```python
from build123d import *

# Parameters (mm, degrees)
F0_W     = 30
F0_H     = 50
F1_DEPTH = 25
F2_W     = 19.697615
F2_H     = 4.146867
F2_W_2   = 19.52483
F2_H_2   = 5.874727
F3_DEPTH = 10
F4_DEPTH = 10
F5_DEPTH = 25
F6_DEPTH = 25
F7_R     = 1.5
F2_R     = 3.544564
F8_DEPTH = 25


with BuildPart() as f1:
    # F0 (on Top) → F1 (new body)
    with BuildSketch(Plane.XY):
        with Locations((40.103809, 0.678835)):
            Rectangle(F0_W, F0_H)
    extrude(amount=F1_DEPTH)

    # F2 (on face) → F3 (join)
    with BuildSketch(Plane.XY.offset(25)):
        with Locations((40.032959, -10.171571)):
            Rectangle(F2_W, F2_H)
        with Locations((40.292139, 12.808978)):
            Rectangle(F2_W_2, F2_H_2)
    extrude(amount=-F3_DEPTH)

    # F2 (on face) → F4 (join)
    with BuildSketch(Plane.XY.offset(25)):
        with Locations((40.292139, 12.808978)):
            Rectangle(F2_W_2, F2_H_2)
        with Locations((40.032959, -10.171571)):
            Rectangle(F2_W, F2_H)
    extrude(amount=-F4_DEPTH)

    # F2 (on face) → F5 (cut)
    with BuildSketch(Plane.XY.offset(25)):
        with Locations((40.292139, 12.808978)):
            Rectangle(F2_W_2, F2_H_2)
    extrude(amount=-F5_DEPTH, mode=Mode.SUBTRACT)

    # F2 (on face) → F6 (cut)
    with BuildSketch(Plane.XY.offset(25)):
        with Locations((40.032959, -10.171571)):
            Rectangle(F2_W, F2_H)
    extrude(amount=-F6_DEPTH, mode=Mode.SUBTRACT)

    # F7
    f7_edges = [f1.edges().sort_by_distance(p)[0] for p in [
        (55.103809, 0.678835, 25),
        (25.103809, 0.678835, 25),
    ]]
    fillet(f7_edges, radius=F7_R)

    # F2 (on face) → F8 (cut)
    with BuildSketch(Plane.XY.offset(25)):
        with Locations((39.648701, 0)):
            Circle(F2_R)
    extrude(amount=-F8_DEPTH, mode=Mode.SUBTRACT)


solid = f1.part
```
Here's how the part is built. I have some questions about the finished solid (model axes, mm). A direction names the side the tool comes from. Round coordinates to 2 decimals unless told otherwise and drop trailing zeros. Order: outer loops, then holes, each group sorted by start corner. A loop starts at its lowest first (then second) coordinate and runs counter-clockwise, first axis right, second up. Notation, with made-up numbers: (-3, 72.25) -> (14, 72.25) arc R25 cw to (14, 96.25) -> close; hole circle Ø3 at (-9.75, -12.5). An arc over 180 degrees is marked (long way). Use a Markdown table: item, result. Add a question column.
(1) Suppose I cut it at B-B, the plane x = 34.25. Please give me the cut outline in (y, z) (3 decimals), and give its area (3 significant figures).
(2) I need wall thicknesses on line 1 along Y through (x, z) = (35, 8.75) (3 decimals); line 2 along Y through (x, z) = (30.25, 23.75) (3 decimals); line 3 along Y through (x, z) = (37.5, 5) (3 decimals). Which ranges of each line are inside material? Lowest first, please.
(3) Suppose I cut it at C-C, the plane z = 15.5. Please give me the cut outline in (x, y) (3 decimals).
(4) For faces 4 (the face through (30.184, -10, 13)), 5 (the face through (40, -24.321, 12)), which set-ups out of +Z, -Z, +X, -X, +Y, -Y let a thin tool reach every point of the face, with its end or its side?
(5) Suppose I cut it at A-A, the plane y = 0. Please give me the cut outline in (x, z), and give its area (3 significant figures).
(6) If we mould it in two halves opening along Y, with no side actions, what happens to faces 1 (the face through (30.53, 13, 13)), 2 (the face through (25.53, 1.03, 24.55)), 3 (the face through (40, 25.679, 12))? For each: released by +Y, released by -Y, zero draft, split by the parting line, or undercut.
Verdict:
| question | item | result |
|---|---|---|
| 1 | outline | (-24.321, 0) -> (-12.245, 0) -> (-12.245, 25) -> (-24.321, 25) -> close; (-8.098, 0) -> (9.872, 0) -> (9.872, 25) -> (-8.098, 25) -> close; (15.746, 0) -> (25.679, 0) -> (25.679, 25) -> (15.746, 25) -> close |
| 1 | area | 999 mm2 |
| 2 | line 1 | -24.321 to -12.245, -8.098 to 9.872, 15.746 to 25.679 |
| 2 | line 2 | -24.321 to -12.245, -8.098 to 25.679 |
| 2 | line 3 | -24.321 to -12.245, -8.098 to -2.819, 2.819 to 9.872, 15.746 to 25.679 |
| 3 | outline | (25.104, -24.321) -> (55.104, -24.321) -> (55.104, 25.679) -> (25.104, 25.679) -> close; hole (30.184, -12.245) -> (49.882, -12.245) -> (49.882, -8.098) -> (30.184, -8.098) -> close; hole (30.53, 9.872) -> (50.055, 9.872) -> (50.055, 15.746) -> (30.53, 15.746) -> close; hole circle Ø7.089 at (39.649, 0) |
| 4 | face 4 | +Z, -Z |
| 4 | face 5 | +Z, -Z, +X, -X, -Y |
| 5 | outline | (25.1, 0) -> (36.1, 0) -> (36.1, 25) -> (26.6, 25) arc R1.5 ccw to (25.1, 23.5) -> close; (43.19, 0) -> (55.1, 0) -> (55.1, 23.5) arc R1.5 ccw to (53.6, 25) -> (43.19, 25) -> close |
| 5 | area | 572 mm2 |
| 6 | face 1 | undercut |
| 6 | face 2 | zero draft |
| 6 | face 3 | released by +Y |
